Model file for the job. Use its own axes, mm. A direction names the side the tool comes from. Give positions to 0.01 mm unless a question says otherwise; leave off trailing zeros. Write each loop counter-clockwise with the first axis right and the second up, starting at its lowest first coordinate (ties: lowest second). Pieces come first, ordered by that corner, then holes.
```python
from build123d import *

# Parameters (mm, degrees)
BOSS_EXTRUDE1_DEPTH = 60
CHAMFER1_SIZE       = 5
SKETCH3_R           = 3
CUT_EXTRUDE1_DEPTH  = 83.462112512


with BuildPart() as part:
    # Sketch2 → Boss-Extrude1 (new body)
    with BuildSketch(Plane(origin=(0, 0, 0), x_dir=(1, 0, 0), z_dir=(0, 1, 0))):
        with BuildLine():
            Line((-20, 20), (20, 20))
            ThreePointArc((20, 20), (40, 0), (20, -20))
            Line((20, -20), (-20, -20))
            ThreePointArc((-20, -20), (-40, 0), (-20, 20))
        make_face()
        with BuildLine():
            Line((7.5, 12.5), (-7.5, 12.5))
            ThreePointArc((-7.5, 12.5), (-20, 0), (-7.5, -12.5))
            Line((-7.5, -12.5), (7.5, -12.5))
            ThreePointArc((7.5, -12.5), (20, 0), (7.5, 12.5))
        make_face(mode=Mode.SUBTRACT)
    extrude(amount=BOSS_EXTRUDE1_DEPTH)

    # Chamfer1
    chamfer1_edges = [part.edges().sort_by_distance(p)[0] for p in [
        (40, 60, 0),
        (0, 60, -20),
        (-40, 60, 0),
        (0, 60, 20),
    ]]
    chamfer(chamfer1_edges, length=CHAMFER1_SIZE)

    # Sketch3 → Cut-Extrude1 (cut, through all)
    with BuildSketch(Plane(origin=(0, 0, -20), x_dir=(-1, 0, 0), z_dir=(0, 0, -1))):
        with Locations((0, 32)):
            Circle(SKETCH3_R)
    extrude(amount=-CUT_EXTRUDE1_DEPTH, mode=Mode.SUBTRACT)


solid = part.part
```
1. Slice it at C-C, the plane y = 40. Write the cut outline in (x, z).
Calculated:
outline: (-20, -20) - (20, -20) arc R20 ccw to (20, 20) - (-20, 20) arc R20 ccw to start; hole (-7.5, -12.5) - (7.5, -12.5) arc R12.5 ccw to (7.5, 12.5) - (-7.5, 12.5) arc R12.5 ccw to start
2. Slice it at B-B, the plane z = 0. Write the cut outline in (x, y).
Calculated:
outline: (-40, 0) - (-20, 0) - (-20, 60) - (-35, 60) - (-40, 55) - close; (20, 0) - (40, 0) - (40, 55) - (35, 60) - (20, 60) - close
3. Which spindle directions (+Z, -Z, +X, -X, +Y, -Y) get a long thin tool onto all of the face, cutting with end or side? Do faces 4 (the flat face through (0, 58, 17)), 5 (the cylindrical face through (20, 30, 0)). Say none if no direction does.
Calculated:
face 4: +Z, +X, -X, +Y
face 5: +Y, -Y
4. Probe probe 1 along Z at (x, y) = (1.5, 36); probe 2 along Y at (x, z) = (0, 15); probe 3 along Y at (x, z) = (0, 17). List the from-to ranges inside material, lowest first.
Calculated:
probe 1: z = -20 to -12.5, 12.5 to 20
probe 2: y = 0 to 29, 35 to 60
probe 3: y = 0 to 29, 35 to 58
5. Pin check, flat tips, straight feed: P1, Ø12, axis at y = 51, z = -5, coming from the +X side; P2, Ø5, axis at y = 43.5, z = -12.5, coming from the -X side. Stop position of each tip, or through.
Calculated:
P1: stops at x = 40
P2: stops at x = -37.32
6. Slice it at A-A, the plane y = 32. Write the cut outline in (x, z).
Calculated:
outline: (-20, -20) - (-3, -20) - (-3, -12.5) - (-7.5, -12.5) arc R12.5 cw to (-7.5, 12.5) - (-3, 12.5) - (-3, 20) - (-20, 20) arc R20 ccw to start; (3, -20) - (20, -20) arc R20 ccw to (20, 20) - (3, 20) - (3, 12.5) - (7.5, 12.5) arc R12.5 cw to (7.5, -12.5) - (3, -12.5) - close
7. Pull direction Y, two halves, no side cores. Call faces 1 (the cylindrical face through (-20, 30, 0)), 2 (the flat face through (0, 60, -14)), 3 (the cylindrical face through (2.21, 34.03, 16.2)): +Y half, -Y half, draft (parallel to the pull), parting line (faces both ways), or undercut.
Calculated:
face 1: draft
face 2: +Y half
face 3: undercut
8. Slice it at D-D, the plane x = 13. Write the cut outline in (y, z), and give its area (3 significant figures).
Calculated:
outline: (0, -20) - (55, -20) - (60, -15) - (60, -11.22) - (0, -11.22) - close; (0, 11.22) - (60, 11.22) - (60, 15) - (55, 20) - (0, 20) - close
area: 1,030 mm2
